from build123d import *

# Parameters (mm, degrees)
F0_W     = 17.3
F0_H     = 14.6
F1_DEPTH = 24


with BuildPart() as f1:
    # F0 (on Front) → F1 (new body)
    with BuildSketch(Plane.XZ):
        Polygon((42.320508, 10), (-7.679492, 10), (-42.320508, -10), (7.679492, -10), align=None)
        Rectangle(F0_W, F0_H, mode=Mode.SUBTRACT)
    extrude(amount=F1_DEPTH)


solid = f1.part
For this review, take the finished solid that the model builds, in its own axes (mm). A direction names the side the tool comes from. Round coordinates to 2 decimals unless told otherwise and drop trailing zeros. Write each loop counter-clockwise with the first axis right and the second up, starting at its lowest first coordinate (ties: lowest second). Pieces come first, ordered by that corner, then holes. Notation, with made-up numbers: M 4,-17.75 L 28,-17.75 A18 cw 28,3.25 Z; hole C -18.5,-30 d11. An arc over 180 degrees is marked long. Write item = value, one per line. Start each with the question number.
(1) The part is to be moulded in two halves that separate along Z. For faces 1 (the face through (0, -12, -7.3)), 2 (the face through (-25, -12, 0)), 3 (the face through (-18, -12, -10)), say which applies: +Z half, -Z half, draft (parallel to the pull), parting line (faces both ways), or undercut.
(2) Clearance check with flat-ended pins moving along their axes: pin 1 Ø5 at (y, z) = (-13, 7.5) entering from -X; pin 2 Ø3 at (y, z) = (-15, 2) entering from +X; pin 3 Ø4 at (y, z) = (-9, -4.5) entering from -X. State where each tip first meets the part, or that it passes through.
(3) We need section C-C (y = -6.5). Give the boundary of the cut face in (x, z).
(4) We need section B-B (z = 2.5). Give the boundary of the cut face in (x, y).
(5) We need section A-A (x = 1). Give the boundary of the cut face in (y, z).
(6) We need section D-D (x = 23). Give the boundary of the cut face in (y, z), then the cut area to 3 significant figures.
(7) For line 1 along Z through (x, y) = (1, -19.75); line 2 along X through (y, z) = (-2, -2.5); line 3 along X through (y, z) = (-22.75, 1.5), list the stretches that pass through material, from the lowest coordinate up.
(8) For faces 4 (the face through (8.65, -12, 0)), 5 (the face through (9, -24, 0)), list the 3-axis set-ups (+Z, -Z, +X, -X, +Y, -Y) from which the entire face can be reached by the end or side of a thin tool; tool diameter is ignored.
Results found:
q1.face_1 = undercut
q1.face_2 = +Z half
q1.face_3 = -Z half
q2.pin_1 = -16.34
q2.pin_2 = 31.06
q2.pin_3 = -36.26
q3.outline = M -42.32,-10 L 7.68,-10 L 42.32,10 L -7.68,10 Z; hole M -8.65,-7.3 L 8.65,-7.3 L 8.65,7.3 L -8.65,7.3 Z
q4.outline = M -20.67,-24 L -8.65,-24 L -8.65,0 L -20.67,0 Z; M 8.65,-24 L 29.33,-24 L 29.33,0 L 8.65,0 Z
q5.outline = M -24,-10 L 0,-10 L 0,-7.3 L -24,-7.3 Z; M -24,7.3 L 0,7.3 L 0,10 L -24,10 Z
q6.outline = M -24,-1.15 L 0,-1.15 L 0,10 L -24,10 Z
q6.area = 268 mm²
q7.line_1 = -10 to -7.3, 7.3 to 10
q7.line_2 = -29.33 to -8.65, 8.65 to 20.67
q7.line_3 = -22.4 to -8.65, 8.65 to 27.6
q8.face_4 = +Y, -Y
q8.face_5 = +Z, -Z, +X, -X, -Y
